The listing builds one solid part. Answer for the finished solid, in the listing's coordinates (mm). Face numbers are marked on the shaded views. Coordinates: 2 decimals unless noted, no trailing zeros. Loops run counter-clockwise (first coordinate to the right, second up) from the corner with the lowest first, then second, coordinate; pieces in that order, holes last. Notation, with made-up numbers: (-28.5, 62) - (28.5, 62) arc R29 cw to (28.5, 99) - close; hole circle Ø11 at (-34.75, -10.5). An arc over 180 degrees is marked (long way). Use one line per item in the form item = value. Start each with the question number.
```python
from build123d import *

# Parameters (mm, degrees)
F0_R      = 5.0419
F1_DEPTH  = 6.35
F2_DEPTH  = 9.525
F4_D      = 3.6576
F5_R      = 1.27
F8_W      = 6.35
F8_H      = 6.35
F9_DEPTH  = 9.5260001
F10_R     = 5.0419
F11_DEPTH = 3.175


with BuildPart() as f1:
    # F0 (on Top) → F1 (new body)
    with BuildSketch(Plane.XY):
        with BuildLine():
            Line((0, 0), (0, 24.13))
            ThreePointArc((0, 24.13), (-9.2620503813, 24.6926494565), (-18.415, 26.2176625565))
            Line((-18.415, 26.2176625565), (-18.415, -32.2023374435))
            add(Edge.make_bspline(
                [(-18.415, -32.2023374435), (-10.35310168, -31.3379440787), (-3.0120759205, -28.1461012273), (0, -24.13)],
                knots=[12.2106695442, 12.2106695442, 12.2106695442, 12.2106695442, 33.2224141479, 33.2224141479, 33.2224141479, 33.2224141479], degree=3))
            Line((0, -24.13), (0, 0))
        make_face()
        with BuildLine():
            Line((-18.415, -32.2023374435), (-18.415, 26.2176625565))
            ThreePointArc((-18.415, 26.2176625565), (-48.7549341061, 39.1874227389), (-72.2748938826, 62.3291118058))
            add(Edge.make_bspline(
                [(-137.9783539955, 35.7469866649), (-73.1067731977, 34.5293954015), (-59.7019699566, 33.2077455579), (-72.2748938826, 62.3291118058)],
                knots=[0, 0, 0, 0, 70.8770346997, 70.8770346997, 70.8770346997, 70.8770346997], degree=3))
            ThreePointArc((-137.9783539955, 35.7469866649), (-162.9147928474, 57.3381501066), (-185.674, 33.4629996115))
            ThreePointArc((-185.674, 33.4629996115), (-180.9856867862, 19.2452424177), (-168.7599080893, 10.6049162859))
            Line((-168.7599080893, 10.6049162859), (-32.4923986546, -31.0562422342))
            add(Edge.make_bspline(
                [(-32.4923986546, -31.0562422342), (-28.0285616621, -32.4209741599), (-23.1000548653, -32.7046670659), (-18.415, -32.2023374435)],
                knots=[0, 0, 0, 0, 12.2106695442, 12.2106695442, 12.2106695442, 12.2106695442], degree=3))
        make_face()
        with Locations((-99.2384759306, 1.0898536678)):
            Circle(F0_R, mode=Mode.SUBTRACT)
        with Locations((-122.5813012408, 8.226471557)):
            Circle(F0_R, mode=Mode.SUBTRACT)
        with Locations((-52.5528253102, -13.1833821107)):
            Circle(F0_R, mode=Mode.SUBTRACT)
        with Locations((-29.21, -20.32)):
            Circle(F0_R, mode=Mode.SUBTRACT)
        with Locations((-75.8956506204, -6.0467642215)):
            Circle(F0_R, mode=Mode.SUBTRACT)
        with Locations((-145.924126551, 15.3630894463)):
            Circle(F0_R, mode=Mode.SUBTRACT)
    extrude(amount=F1_DEPTH)

    # F0 (on Top) → F2 (join)
    with BuildSketch(Plane.XY):
        with BuildLine():
            Line((-18.415, -32.2023374435), (-18.415, 26.2176625565))
            ThreePointArc((-18.415, 26.2176625565), (-48.7549341061, 39.1874227389), (-72.2748938826, 62.3291118058))
            add(Edge.make_bspline(
                [(-137.9783539955, 35.7469866649), (-73.1067731977, 34.5293954015), (-59.7019699566, 33.2077455579), (-72.2748938826, 62.3291118058)],
                knots=[0, 0, 0, 0, 70.8770346997, 70.8770346997, 70.8770346997, 70.8770346997], degree=3))
            ThreePointArc((-137.9783539955, 35.7469866649), (-162.9147928474, 57.3381501066), (-185.674, 33.4629996115))
            ThreePointArc((-185.674, 33.4629996115), (-180.9856867862, 19.2452424177), (-168.7599080893, 10.6049162859))
            Line((-168.7599080893, 10.6049162859), (-32.4923986546, -31.0562422342))
            add(Edge.make_bspline(
                [(-32.4923986546, -31.0562422342), (-28.0285616621, -32.4209741599), (-23.1000548653, -32.7046670659), (-18.415, -32.2023374435)],
                knots=[0, 0, 0, 0, 12.2106695442, 12.2106695442, 12.2106695442, 12.2106695442], degree=3))
        make_face()
        with Locations((-99.2384759306, 1.0898536678)):
            Circle(F0_R, mode=Mode.SUBTRACT)
        with Locations((-122.5813012408, 8.226471557)):
            Circle(F0_R, mode=Mode.SUBTRACT)
        with Locations((-52.5528253102, -13.1833821107)):
            Circle(F0_R, mode=Mode.SUBTRACT)
        with Locations((-29.21, -20.32)):
            Circle(F0_R, mode=Mode.SUBTRACT)
        with Locations((-75.8956506204, -6.0467642215)):
            Circle(F0_R, mode=Mode.SUBTRACT)
        with Locations((-145.924126551, 15.3630894463)):
            Circle(F0_R, mode=Mode.SUBTRACT)
    extrude(amount=F2_DEPTH)

    # F4 (through all)
    with Locations(Plane.XY.offset(6.35)):
        with Locations((-12.065, 16.0576625565), (-12.065, 3.3576625565), (-12.065, -9.3423374435), (-12.065, -22.0423374435)):
            Hole(F4_D / 2)

    # F5
    f5_edges = [f1.edges().sort_by_distance(p)[0] for p in [
        (-72.274894, 62.329112, 3.175),
        (-72.274894, 62.329112, 7.9375),
    ]]
    fillet(f5_edges, radius=F5_R)

    # F8 (on Top) → F9 (cut, through all)
    with BuildSketch(Plane.XY):
        with Locations((-52.5528253102, 7.1366178893)):
            Rectangle(F8_W, F8_H)
    extrude(amount=F9_DEPTH, mode=Mode.SUBTRACT)

    # F10 (on face) → F11 (join)
    with BuildSketch(Plane(origin=(0, 0, 0), x_dir=(1, 0, 0), z_dir=(0, 0, -1))):
        with BuildLine():
            ThreePointArc((-29.21, 12.1031), (-23.3997742897, 14.5097742897), (-20.9931, 20.32))
            ThreePointArc((-20.9931, 20.32), (-29.21, 28.5369), (-37.4269, 20.32))
            ThreePointArc((-37.4269, 20.32), (-35.0202257103, 14.5097742897), (-29.21, 12.1031))
        make_face()
        with Locations((-29.21, 20.32)):
            Circle(F10_R, mode=Mode.SUBTRACT)
        with BuildLine():
            ThreePointArc((-29.21, 12.1031), (-35.0202257103, 14.5097742897), (-37.4269, 20.32))
            Line((-37.4269, 20.32), (-37.4269, 12.1031))
            Line((-37.4269, 12.1031), (-29.21, 12.1031))
        make_face()
        with BuildLine():
            ThreePointArc((-52.5528253102, 4.9664821107), (-58.3630510205, 7.3731564004), (-60.7697253102, 13.1833821107))
            Line((-60.7697253102, 13.1833821107), (-60.7697253102, 4.9664821107))
            Line((-60.7697253102, 4.9664821107), (-52.5528253102, 4.9664821107))
        make_face()
        with BuildLine():
            ThreePointArc((-44.3359253102, 13.1833821107), (-52.5528253102, 21.4002821107), (-60.7697253102, 13.1833821107))
            ThreePointArc((-60.7697253102, 13.1833821107), (-58.3630510205, 7.3731564004), (-52.5528253102, 4.9664821107))
            ThreePointArc((-52.5528253102, 4.9664821107), (-46.7425995999, 7.3731564004), (-44.3359253102, 13.1833821107))
        make_face()
        with Locations((-52.5528253102, 13.1833821107)):
            Circle(F10_R, mode=Mode.SUBTRACT)
        with BuildLine():
            ThreePointArc((-75.8956506204, -2.1701357785), (-81.7058763307, 0.2365385111), (-84.1125506204, 6.0467642215))
            Line((-84.1125506204, 6.0467642215), (-84.1125506204, -2.1701357785))
            Line((-84.1125506204, -2.1701357785), (-75.8956506204, -2.1701357785))
        make_face()
        with BuildLine():
            ThreePointArc((-67.6787506204, 6.0467642215), (-75.8956506204, 14.2636642215), (-84.1125506204, 6.0467642215))
            ThreePointArc((-84.1125506204, 6.0467642215), (-81.7058763307, 0.2365385111), (-75.8956506204, -2.1701357785))
            ThreePointArc((-75.8956506204, -2.1701357785), (-70.0854249101, 0.2365385111), (-67.6787506204, 6.0467642215))
        make_face()
        with Locations((-75.8956506204, 6.0467642215)):
            Circle(F10_R, mode=Mode.SUBTRACT)
        with BuildLine():
            ThreePointArc((-99.2384759306, -9.3067536678), (-105.0487016409, -6.9000793781), (-107.4553759306, -1.0898536678))
            Line((-107.4553759306, -1.0898536678), (-107.4553759306, -9.3067536678))
            Line((-107.4553759306, -9.3067536678), (-99.2384759306, -9.3067536678))
        make_face()
        with BuildLine():
            ThreePointArc((-91.0215759306, -1.0898536678), (-99.2384759306, 7.1270463322), (-107.4553759306, -1.0898536678))
            ThreePointArc((-107.4553759306, -1.0898536678), (-105.0487016409, -6.9000793781), (-99.2384759306, -9.3067536678))
            ThreePointArc((-99.2384759306, -9.3067536678), (-93.4282502203, -6.9000793781), (-91.0215759306, -1.0898536678))
        make_face()
        with Locations((-99.2384759306, -1.0898536678)):
            Circle(F10_R, mode=Mode.SUBTRACT)
        with BuildLine():
            ThreePointArc((-122.5813012408, -16.443371557), (-128.3915269511, -14.0366972674), (-130.7982012408, -8.226471557))
            Line((-130.7982012408, -8.226471557), (-130.7982012408, -16.443371557))
            Line((-130.7982012408, -16.443371557), (-122.5813012408, -16.443371557))
        make_face()
        with BuildLine():
            ThreePointArc((-114.3644012408, -8.226471557), (-122.5813012408, -0.009571557), (-130.7982012408, -8.226471557))
            ThreePointArc((-130.7982012408, -8.226471557), (-128.3915269511, -14.0366972674), (-122.5813012408, -16.443371557))
            ThreePointArc((-122.5813012408, -16.443371557), (-116.7710755305, -14.0366972674), (-114.3644012408, -8.226471557))
        make_face()
        with Locations((-122.5813012408, -8.226471557)):
            Circle(F10_R, mode=Mode.SUBTRACT)
        with BuildLine():
            ThreePointArc((-145.924126551, -23.5799894463), (-151.7343522614, -21.1733151566), (-154.141026551, -15.3630894463))
            Line((-154.141026551, -15.3630894463), (-154.141026551, -23.5799894463))
            Line((-154.141026551, -23.5799894463), (-145.924126551, -23.5799894463))
        make_face()
        with BuildLine():
            ThreePointArc((-137.707226551, -15.3630894463), (-145.924126551, -7.1461894463), (-154.141026551, -15.3630894463))
            ThreePointArc((-154.141026551, -15.3630894463), (-151.7343522614, -21.1733151566), (-145.924126551, -23.5799894463))
            ThreePointArc((-145.924126551, -23.5799894463), (-140.1139008407, -21.1733151566), (-137.707226551, -15.3630894463))
        make_face()
        with Locations((-145.924126551, -15.3630894463)):
            Circle(F10_R, mode=Mode.SUBTRACT)
    extrude(amount=F11_DEPTH)


solid = f1.part
```
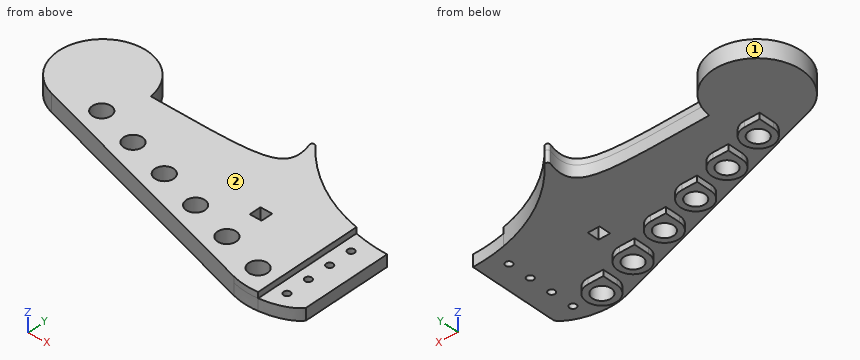
(1) A cutting plane is placed at A-A (x = -160). Determine the outline of the cut face in (y, z) (3 decimals), then the cut area to 3 significant figures.
(2) Find the intervals of material crossed by probe 1 along X at (y, z) = (12, 6.75) (1 decimal); probe 2 along Z at (x, y) = (-72, 9.5) (3 decimals); probe 3 along Y at (x, z) = (-142.5, -0.75), in increasing order. Write a range as from..to.
(3) Determine the mould class of the marked faces 1 and 2 for opening direction X: +X half, -X half, draft (parallel to the pull), parting line (faces both ways), or undercut.
(4) Each of these flat-tipped pins is pushed along its axis until it touches: pin 1 Ø3 at (x, z) = (-52, 3.5) entering from +Y; pin 2 Ø4 at (x, y) = (-12.06, -9.34) entering from -Z; pin 3 Ø4 at (x, z) = (-162, 8) entering from -Y; pin 4 Ø3 at (x, y) = (-12.06, 16.06) entering from -Z. Where does it stop, or does it pass through?
Evaluation:
q1.outline = (7.927, 0) - (57.3, 0) - (57.3, 9.525) - (7.927, 9.525) - close
q1.area = 470 mm^2
q2.probe_1 = -172.3..-149.7, -142.2..-125.9, -119.2..-18.4
q2.probe_2 = 0..9.525
q2.probe_3 = 7.89..11.66, 19.06..22.83
q3.face_1 = undercut
q3.face_2 = draft
q4.pin_1 = 42.6
q4.pin_2 = 0
q4.pin_3 = 7.93
q4.pin_4 = through
